Autodesk Fusion 360 part; units mm, degrees
sketch "Sketch1" plane through (0, 0, 0) normal (0, 0, 1) x (1, 0, 0)
  line L0 (20, -10) -> (-20, -10)
  line L1 (-20, -10) -> (-20, 10)
  line L2 (-20, 10) -> (20, 10)
  line L3 (20, 10) -> (20, -10)
  line L4 (20, -10) -> (-20, 10) construction
  line L5 (-20, -10) -> (20, 10) construction
  line L6 (22.5, -12.5) -> (-22.5, -12.5)
  line L7 (-22.5, -12.5) -> (-22.5, 12.5)
  line L8 (-22.5, 12.5) -> (22.5, 12.5)
  line L9 (22.5, 12.5) -> (22.5, -12.5)
  line L10 (22.5, -12.5) -> (-22.5, 12.5) construction
  line L11 (-22.5, -12.5) -> (22.5, 12.5) construction
  dimension "d1" = 40
  dimension "d2" = 20
  dimension "d3" = 45
  dimension "d4" = 25
extrude "Extrude1" add sketch "Sketch1" along normal blind 11 makes body 1
sketch "Sketch4" plane through (22.5, 0, 0) normal (1, 0, 0) x (0, 1, 0)
  line L0 (-12.5, 0) -> (12.5, 0)
  line L1 (12.5, 0) -> (12.5, 11)
  line L2 (12.5, 11) -> (-12.5, 11)
  line L3 (-12.5, 11) -> (-12.5, 0)
  line L4 (-12.5, 0) -> (12.281, 0) construction
  line L5 (-12.5, 0) -> (-20, -25)
  line L6 (-20, -25) -> (20, -25)
  line L7 (20, -25) -> (12.5, 0)
  line L8 (12.5, 0) -> (20, -25) construction
  line L9 (12.281, -0.0657) -> (12.5, 0) construction
  line L10 (-12.5, 0) -> (-20, -25) construction
  line L11 (17.0904, -24.0014) -> (10.4521, -1.8738)
  line L12 (-17.0895, -23.9987) -> (-10.4636, -1.8738) construction
  line L13 (-1, -1.8738) -> (-1, -24)
  line L14 (1, -24.0002) -> (1, -1.8738)
  line L15 (-17.0895, -23.9987) -> (-1, -24)
  line L16 (1, -24.0002) -> (17.0904, -24.0014)
  line L17 (17.0904, -24.0014) -> (10.4521, -1.8738) construction
  line L18 (9.8899, 0) -> (9.2425, 2.1581) construction
  line L19 (-17.0895, -23.9987) -> (-10.4636, -1.8738)
  line L20 (-10.4636, -1.8738) -> (-1, -1.8738)
  line L21 (1, -1.8738) -> (10.4521, -1.8738)
extrude "Extrude10" add sketch "Sketch4" against normal blind 2 separate body contours L11 L14 L16 L21 | L13 L15 L19 L20 makes body 2 at (22.5, 9.5141, -16.6251) makes body 3 at (22.5, -9.5177, -16.6242)
extrude "Extrude8" add sketch "Sketch4" against normal up to surface (45 mm away) contours L0 L5 L6 L7 bodies 1
sketch "Sketch9" plane through (0, 0, -1.8738) normal (0, 0, -1) x (1, 0, 0)
  line L0 (-22.5, 10.4636) -> (-22.5, 1)
  line L1 (-22.5, 1) -> (22.5, 1)
  line L2 (22.5, 1) -> (22.5, 10.4636)
  line L3 (22.5, 10.4636) -> (-22.5, 10.4636)
  line L4 (-1, 20) -> (1, 20)
  line L5 (1, 20) -> (1, -20)
  line L6 (1, -20) -> (-1, -20)
  line L7 (-1, -20) -> (-1, 20)
  line L8 (-22.5, 19) -> (-21.5, 20)
  line L9 (-21.5, 20) -> (-2, 0.5)
  line L10 (-2, 0.5) -> (-3, -0.5)
  line L11 (-3, -0.5) -> (-22.5, 19)
  line L12 (-22.5, -19) -> (-21.5, -20)
  line L13 (-21.5, -20) -> (-2, -0.5)
  line L14 (-2, -0.5) -> (-3, 0.5)
  line L15 (-3, 0.5) -> (-22.5, -19)
  line L16 (22.5, -19) -> (21.5, -20)
  line L17 (21.5, -20) -> (1.9964, -0.4964)
  line L18 (1.9964, -0.4964) -> (2.9964, 0.5036)
  line L19 (2.9964, 0.5036) -> (22.5, -19)
  line L20 (21.5, 20) -> (22.5, 19)
  line L21 (22.5, 19) -> (2.5, -1)
  line L22 (2.5, -1) -> (1.5, 0)
  line L23 (1.5, 0) -> (21.5, 20)
extrude "Extrude9" add sketch "Sketch9" along normal up to surface (23.1262 mm away) contours L3 L8 L9 L11 | L1 L3 L9 L11 | L1 L9 L10 L11 L14 L15 | L10 L11 L14 L15 | L10 L11 L12 L13 L14 L15 | L3 L4 L5 L7 | L1 L3 L5 L7 | L1 L5 L6 L7 | L3 L20 L21 L23 | L1 L3 L21 L23 | L1 L18 L19 L21 L22 L23 | L17 L18 L19 L21 L22 | L16 L17 L19 L21 bodies 1
sketch "Sketch10" plane through (-22.5, 0, 0) normal (-1, 0, 0) x (0, -1, 0)
  line L0 (-1, -1.8738) -> (-1, -24.0002)
  line L1 (-1, -24.0002) -> (-17.0904, -24.0014)
  line L2 (-17.0904, -24.0014) -> (-10.4521, -1.8738)
  line L3 (-10.4521, -1.8738) -> (-1, -1.8738)
  line L4 (10.4636, -1.8738) -> (17.0895, -23.9987)
  line L5 (17.0895, -23.9987) -> (1, -24)
  line L6 (1, -24) -> (1, -1.8738)
  line L7 (1, -1.8738) -> (10.4636, -1.8738)
  line L8 (-19, -21.6667) -> (-20, -25)
  line L9 (-20, -25) -> (20, -25)
  line L10 (20, -25) -> (19, -21.6667)
  line L11 (19, -21.6667) -> (12.5, 0)
  line L12 (12.5, 0) -> (12.5, 11)
  line L13 (12.5, 11) -> (-12.5, 11)
  line L14 (-12.5, 11) -> (-12.5, 0)
  line L15 (-12.5, 0) -> (-19, -21.6667)
  line L16 (-25.8354, 18.4889) -> (28, 18.4889)
  line L17 (28, 18.4889) -> (28, -29)
  line L18 (28, -29) -> (-25.8354, -29)
  line L19 (-25.8354, -29) -> (-25.8354, 18.4889)
extrude "Extrude12" cut sketch "Sketch10" against normal blind 74 contours L16 L17 L18 L19 bodies 1
extrude "Extrude11" add sketch "Sketch10" against normal blind 2 contours L0 L1 L2 L3 | L4 L5 L6 L7 bodies 1
combine "Combine2" operation add target body 1 tool bodies 2 3
equation "d3 = 40 mm + 5 mm"
equation "d4 = 20 mm + 5 mm"
Work out the finished part from the listing and answer in its coordinate system (mm). A direction names the side the tool comes from. Give positions to 0.01 mm unless a question says otherwise; leave off trailing zeros. Loops run counter-clockwise (first coordinate to the right, second up) from the corner with the lowest first, then second, coordinate; pieces in that order, holes last. Notation, with made-up numbers: M -27.5,65.5 L -13.5,65.5 A16 ccw -13.5,82.5 Z; hole C -7.5,0.25 d11. An arc over 180 degrees is marked long. Use CSV: the item, a comma, the result in double quotes.
1) Find section D-D on z = -9. Give the number of separate pieces and of enclosed holes in the cut face, plus the area to 3 significant figures.
Answer:
separate pieces,"1"
enclosed holes,"8"
area,"556 mm^2"
2) Which of the six approach directions +Z, -Z, +X, -X, +Y, -Y give full straight-line access (tool end or side, diameter ignored) to faces 1 (the flat face through (0, -10, 5)), 2 (the flat face through (-18.635, 12.317, -8.089))?
Answer:
face 1,"+Z"
face 2,"none"
3) Given P1, Ø17.5, axis at x = -10.5, z = -15.5, coming from the +Y side (3 decimals); P2, Ø13, axis at x = 11, z = -12.5, coming from the -Y side; P3, Ø9, axis at x = -3, z = 4, coming from the -Y side, each flat-ended and moving along its own axis, determine where each tip first touches the part or whether it passes through.
Answer:
P1,"y = 19.775"
P2,"y = -18.2"
P3,"y = -12.65"
4) Consider L1, parallel to Z at x = -17, y = 6; L2, parallel to Y at x = -7, z = 6; L3, parallel to Y at x = -12.5, z = -14.5. Determine where each line is inside the solid, lowest interval first.
Answer:
L1,"-25 to -24, -1.87 to 0"
L2,"-12.5 to -10, 10 to 12.5"
L3,"-16.85 to -14.24, -11 to -9, -1 to 1, 9 to 11, 14.24 to 16.85"
5) Find section A-A on z = 8.5. Write down the section's boundary in (x, y).
Answer:
outline,"M -22.5,-12.5 L 22.5,-12.5 L 22.5,12.5 L -22.5,12.5 Z; hole M -20,-10 L 20,-10 L 20,10 L -20,10 Z"
6) Find section B-B on y = -14. Write down the section's boundary in (x, z), plus the area to 3 significant figures.
Answer:
outline,"M -22.5,-25 L 22.5,-25 L 22.5,-5 L 17.5,-5 L -15.5,-5 L -22.5,-5 Z; hole M -20.5,-24 L -17.5,-24 L -17.5,-13.68 L -20.5,-13.68 Z; hole M -15.5,-24 L -1,-24 L -1,-13.68 L -15.5,-13.68 Z; hole M 1,-24 L 15.5,-24 L 15.5,-13.68 L 1,-13.68 Z; hole M 17.5,-24 L 20.5,-24 L 20.5,-13.68 L 17.5,-13.68 Z"
area,"539 mm^2"
7) Find section C-C on x = -9. Write down the section's boundary in (y, z), plus the area to 3 significant figures.
Answer:
outline,"M -20,-25 L 20,-25 L 12.5,0 L 12.5,11 L 10,11 L 10,0 L -10,0 L -10,11 L -12.5,11 L -12.5,0 Z; hole M -17.09,-24 L -7.5,-24 L -7.5,-1.87 L -10.46,-1.87 Z; hole M -5.5,-24 L -1,-24 L -1,-1.87 L -5.5,-1.87 Z; hole M 1,-24 L 5.5,-24 L 5.5,-1.87 L 1,-1.87 Z; hole M 7.5,-24 L 17.09,-24 L 10.45,-1.87 L 7.5,-1.87 Z"
area,"391 mm^2"
8) Determine the mould class of faces 3 (the flat face through (-20.5, 7, -13)), 4 (the flat face through (0, 10, 5)), 5 (the flat face through (0, 0, -25)) for opening direction Y: released by +Y, released by -Y, zero draft, split by the parting line, or undercut.
Answer:
face 3,"undercut"
face 4,"undercut"
face 5,"zero draft"
